```python
from build123d import *

# Parameters (mm, degrees)
ESQUISSE2_R             = 4
EXTRUSION1_DEPTH        = 8.5
ESQUISSE3_R             = 6
EXTRUSION2_DEPTH        = 2
ESQUISSE4_R             = 2
ENL_V_MAT_EXTRU_1_DEPTH = 11.5
ENL_V_MAT_EXTRU_2_DEPTH = 5.5
CHANFREIN1_SIZE         = 0.3
CHANFREIN2_SIZE         = 1


with BuildPart() as part:
    # Esquisse2 → Extrusion1 (new body)
    with BuildSketch(Plane(origin=(0, 0, 0), x_dir=(1, 0, 0), z_dir=(0, 1, 0))):
        with Locations(Location((0, 0, 0), (0, 0, 270))):  # turned: the seam where the file's is
            Circle(ESQUISSE2_R)
    extrude(amount=-EXTRUSION1_DEPTH)

    # Esquisse3 → Extrusion2 (add)
    with BuildSketch(Plane(origin=(0, 0, 0), x_dir=(-1, 0, 0), z_dir=(0, 1, 0))):
        with Locations(Location((0, 0, 0), (0, 0, 90))):  # turned: the seam where the file's is
            Circle(ESQUISSE3_R)
    extrude(amount=EXTRUSION2_DEPTH)

    # Esquisse4 → Enlèv. mat.-Extru.1 (cut, through all)
    with BuildSketch(Plane(origin=(0, 2, 0), x_dir=(-1, 0, 0), z_dir=(0, 1, 0))):
        with Locations(Location((0, 0, 0), (0, 0, 90))):  # turned: the seam where the file's is
            Circle(ESQUISSE4_R)
    extrude(amount=-ENL_V_MAT_EXTRU_1_DEPTH, mode=Mode.SUBTRACT)

    # Esquisse5 → Enlèv. mat.-Extru.2 (cut)
    with BuildSketch(Plane(origin=(0, 2, 0), x_dir=(-1, 0, 0), z_dir=(0, 1, 0))):
        Polygon((0, -2.886751346), (2.5, -1.443375673), (2.5, 1.443375673), (0, 2.886751346), (-2.5, 1.443375673), (-2.5, -1.443375673), align=None)
    extrude(amount=-ENL_V_MAT_EXTRU_2_DEPTH, mode=Mode.SUBTRACT)

    # Chanfrein1
    chanfrein1_edges = [part.edges().sort_by_distance(p)[0] for p in [
        (0, 0, -6),
        (0, 2, -6),
    ]]
    chamfer(chanfrein1_edges, length=CHANFREIN1_SIZE)

    # Chanfrein2
    chanfrein2_edges = [part.edges().sort_by_distance(p)[0] for p in [
        (0, -8.5, -4),
    ]]
    chamfer(chanfrein2_edges, length=CHANFREIN2_SIZE)


solid = part.part
```
Could you check a few things on this model? Use its own coordinates, in mm. A direction names the side the tool comes from. Round coordinates to 2 decimals unless told otherwise and drop trailing zeros. Write each loop counter-clockwise with the first axis right and the second up, starting at its lowest first coordinate (ties: lowest second). Pieces come first, ordered by that corner, then holes. Notation, with made-up numbers: M -35.75,-2 L 20.25,-2 A20 cw 20.25,14 Z; hole C -4,55 d1. An arc over 180 degrees is marked long. Answer in a Markdown table with one row per item. Add a question column.
Q1. Imagine slicing it at C-C (y = -4). Please give me the cut outline in (x, z), then the cut area to 3 significant figures.
Q2. If we mould it in two halves opening along Z, with no side actions, what happens to faces 1 (the flat face through (-4, 0, 2)), 2 (the cylindrical face through (-3.905, -3.698, -0.867)), 3 (the flat face through (-1.233, -0.712, -2.175)), 4 (the cylindrical face through (-2, -6, 0))? For each: +Z half, -Z half, draft (parallel to the pull), parting line (faces both ways), or undercut.
Q3. Imagine slicing it at A-A (z = 0). Please give me the cut outline in (x, y), then the cut area to 3 significant figures.
Q4. Will these pins go through, and if not, where does the flat tip stop? pin 1 Ø5 at (y, z) = (-1.5, -4.5) entering from +X; pin 2 Ø5 at (x, y) = (2, -4) entering from +Z; pin 3 Ø3 at (y, z) = (-2, 0.5) entering from -X.
Q5. On a 3-axis mill with a long thin cutter (end or side, diameter ignored), from which of +Z, -Z, +X, -X, +Y, -Y can I reach the whole of each face in a straight line? I mean faces 5 (the flat face through (1, -3.5, -2)), 6 (the flat face through (-1, -8.5, 2)). Say none if no direction works.
Q6. If I drill on line 1 (X direction, y = -4.9, z = 0); line 2 (Y direction, x = 2.25, z = -0.5); line 3 (Y direction, x = 2.75, z = 4.5), over which ranges is the centre line in solid material (lowest first)? Write a range as from..to.
Q7. Imagine slicing it at B-B (y = -2.25). Please give me the cut outline in (x, z), then the cut area to 3 significant figures.
Values:
| question | item | result |
|---|---|---|
| 1 | outline | C 0,0 d8; hole C 0,0 d4 |
| 1 | area | 37.7 mm^2 |
| 2 | face 1 | draft |
| 2 | face 2 | parting line |
| 2 | face 3 | undercut |
| 2 | face 4 | undercut |
| 3 | outline | M -6,0.3 L -5.7,0 L -4,0 L -4,-7.5 L -3,-8.5 L -2,-8.5 L -2,-3.5 L -2.5,-3.5 L -2.5,2 L -5.7,2 L -6,1.7 Z; M 2,-8.5 L 3,-8.5 L 4,-7.5 L 4,0 L 5.7,0 L 6,0.3 L 6,1.7 L 5.7,2 L 2.5,2 L 2.5,-3.5 L 2,-3.5 Z |
| 3 | area | 43.3 mm^2 |
| 4 | pin 1 | x = 5.32 |
| 4 | pin 2 | z = 4 |
| 4 | pin 3 | x = -4 |
| 5 | face 5 | +Y |
| 5 | face 6 | +Z, -Z, +X, -X, -Y |
| 6 | line 1 | -4..-2, 2..4 |
| 6 | line 2 | -8.5..-3.5 |
| 6 | line 3 | 0..2 |
| 7 | outline | C 0,0 d8; hole M -2.5,-1.44 L 0,-2.89 L 2.5,-1.44 L 2.5,1.44 L 0,2.89 L -2.5,1.44 Z |
| 7 | area | 28.6 mm^2 |
